```python
from build123d import *

# Parameters (mm, degrees)
SKETCH1_R           = 2
SKETCH1_R_2         = 1.9
SKETCH1_R_3         = 2.5
BOSS_EXTRUDE1_DEPTH = 5


with BuildPart() as part:
    # Sketch1 → Boss-Extrude1 (new body)
    with BuildSketch(Plane.XY):
        with BuildLine():
            Line((-55, 45), (-55, -45))
            ThreePointArc((-55, -45), (-54.267766953, -46.767766953), (-52.5, -47.5))
            Line((-52.5, -47.5), (57, -47.5))
            ThreePointArc((57, -47.5), (58.767766953, -46.767766953), (59.5, -45))
            Line((59.5, -45), (59.5, -10.5))
            ThreePointArc((59.5, -10.5), (58.767766953, -8.732233047), (57, -8))
            Line((57, -8), (22, -8))
            ThreePointArc((22, -8), (14, 0), (22, 8))
            Line((22, 8), (57, 8))
            ThreePointArc((57, 8), (58.767766953, 8.732233047), (59.5, 10.5))
            Line((59.5, 10.5), (59.5, 45))
            ThreePointArc((59.5, 45), (58.767766953, 46.767766953), (57, 47.5))
            Line((57, 47.5), (-52.5, 47.5))
            ThreePointArc((-52.5, 47.5), (-54.267766953, 46.767766953), (-55, 45))
        make_face()
        with Locations(Location((15.562803405, 24, 0), (0, 0, 180))):
            Circle(SKETCH1_R, mode=Mode.SUBTRACT)
        with Locations((22, -14.25)):
            Circle(SKETCH1_R_2, mode=Mode.SUBTRACT)
        with Locations(Location((22, 14.25, 0), (0, 0, 180))):
            Circle(SKETCH1_R_2, mode=Mode.SUBTRACT)
        with Locations((52, -40)):
            Circle(SKETCH1_R_3, mode=Mode.SUBTRACT)
        with Locations((-47.5, -40)):
            Circle(SKETCH1_R_3, mode=Mode.SUBTRACT)
        with Locations((15.562803405, -24)):
            Circle(SKETCH1_R, mode=Mode.SUBTRACT)
        with Locations((-17.5, 0)):
            Circle(SKETCH1_R, mode=Mode.SUBTRACT)
        with Locations(Location((-47.5, 40, 0), (0, 0, 180))):
            Circle(SKETCH1_R_3, mode=Mode.SUBTRACT)
        with Locations(Location((52, 40, 0), (0, 0, 180))):
            Circle(SKETCH1_R_3, mode=Mode.SUBTRACT)
    extrude(amount=BOSS_EXTRUDE1_DEPTH)


solid = part.part
```
Geometry check sheet. Reference: the model listing, model coordinates, mm. A direction names the side the tool comes from. Round coordinates to 2 decimals unless told otherwise and drop trailing zeros. Order: outer loops, then holes, each group sorted by start corner. A loop starts at its lowest first (then second) coordinate and runs counter-clockwise, first axis right, second up. Notation, with made-up numbers: (-3, 44) - (32, 44) arc R20 ccw to (32, 62) - close; hole circle Ø10 at (45, -13.5). An arc over 180 degrees is marked (long way). Use a Markdown table: item, result. Add a question column.
(1) Sectioned sample at B-B, the plane y = 0. Enter the section's corners in (x, z).
(2) Sectioned sample at D-D, the plane y = 40. Enter the section's corners in (x, z), and give its area (4 significant figures).
(3) Sectioned sample at C-C, the plane z = 3.75. Count the separate pieces of the cut face and the enclosed holes in it, and give its area (3 significant figures).
(4) Tool access check on faces 1 (the cylindrical face through (20.6, -12.966, 2.465)), 2 (the cylindrical face through (59, 9, 2)). Record the directions out of +Z, -Z, +X, -X, +Y, -Y that give a thin tool (end or side, any length) a straight path to the whole face; none if there is none.
(5) Depth check by flat-ended pin: pin 1 (3 mm diameter, centred on x = 15.56, y = -24, fed in from -Z). Enter the tip coordinate at first touch or a pass-through.
(6) Release check for a two-part mould opening along Y. For faces 3 (the flat face through (-55, 1, 2)), 4 (the cylindrical face through (16.638, -22.314, 2.465)), 5 (the cylindrical face through (58.748, -46.787, 2.465)) record: pulls with the +Y half, pulls with the -Y half, needs draft (parallel to the pull), parting line crosses it, or undercut.
(7) Material ranges on line 1 along Y through (x, z) = (52, 2.9); line 2 along Y through (x, z) = (22, 3.85); line 3 along Y through (x, z) = (-47.5, 1.05), recorded low to high. Write a range as [from, to].
(8) Sectioned sample at A-A, the plane x = 29. Enter the section's corners in (y, z).
Answers below:
| question | item | result |
|---|---|---|
| 1 | outline | (-55, 0) - (-19.5, 0) - (-19.5, 5) - (-55, 5) - close; (-15.5, 0) - (14, 0) - (14, 5) - (-15.5, 5) - close |
| 2 | outline | (-55, 0) - (-50, 0) - (-50, 5) - (-55, 5) - close; (-45, 0) - (49.5, 0) - (49.5, 5) - (-45, 5) - close; (54.5, 0) - (59.5, 0) - (59.5, 5) - (54.5, 5) - close |
| 2 | area | 522.5 mm² |
| 3 | separate pieces | 1 |
| 3 | enclosed holes | 9 |
| 3 | area | 10,000 mm² |
| 4 | face 1 | +Z, -Z |
| 4 | face 2 | +Z, -Z, +X |
| 5 | pin 1 | through |
| 6 | face 3 | needs draft |
| 6 | face 4 | undercut |
| 6 | face 5 | pulls with the -Y half |
| 7 | line 1 | [-47.5, -42.5], [-37.5, -8], [8, 37.5], [42.5, 47.5] |
| 7 | line 2 | [-47.5, -16.15], [-12.35, -8], [8, 12.35], [16.15, 47.5] |
| 7 | line 3 | [-47.5, -42.5], [-37.5, 37.5], [42.5, 47.5] |
| 8 | outline | (-47.5, 0) - (-8, 0) - (-8, 5) - (-47.5, 5) - close; (8, 0) - (47.5, 0) - (47.5, 5) - (8, 5) - close |
